Can you work these out from the model? Positions are in its coordinate system, mm. Round coordinates to 2 decimals unless told otherwise and drop trailing zeros. Order: outer loops, then holes, each group sorted by start corner. A loop starts at its lowest first (then second) coordinate and runs counter-clockwise, first axis right, second up. Notation, with made-up numbers: (64, 78) - (106, 78) arc R16 cw to (106, 99) - close; hole circle Ø10 at (34, 35.5). An arc over 180 degrees is marked (long way). Write item = value, one per line.
from build123d import *

# Parameters (mm, degrees)
ESBO_O1_W                = 250
ESBO_O1_H                = 130
RESSALTO_EXTRUS_O1_DEPTH = 6
FILETE1_R                = 50
ESBO_O2_R                = 2
CORTE_EXTRUS_O1_DEPTH    = 6
ESBO_O3_R                = 2.1
CORTE_EXTRUS_O2_DEPTH    = 6
ESBO_O4_R                = 2
CORTE_EXTRUS_O3_DEPTH    = 6
CHANFRO1_SIZE            = 2.3


with BuildPart() as part:
    # Esboço1 → Ressalto-extrusão1 (new body)
    with BuildSketch(Plane.XY):
        Rectangle(ESBO_O1_W, ESBO_O1_H)
    extrude(amount=RESSALTO_EXTRUS_O1_DEPTH)

    # Filete1
    filete1_edges = [part.edges().sort_by_distance(p)[0] for p in [
        (-125, 65, 3),
    ]]
    fillet(filete1_edges, radius=FILETE1_R)

    # Esboço2 → Corte-extrusão1 (cut)
    with BuildSketch(Plane(origin=(0, 0, 0), x_dir=(-1, 0, 0), z_dir=(0, 0, -1))):
        with Locations((0, -55)):
            Circle(ESBO_O2_R)
        with Locations((105, -55)):
            Circle(ESBO_O2_R)
        with Locations((-105, -55)):
            Circle(ESBO_O2_R)
    extrude(amount=-CORTE_EXTRUS_O1_DEPTH, mode=Mode.SUBTRACT)

    # Esboço3 → Corte-extrusão2 (cut)
    with BuildSketch(Plane(origin=(0, 0, 0), x_dir=(-1, 0, 0), z_dir=(0, 0, -1))):
        with Locations((-70, 55)):
            Circle(ESBO_O3_R)
        with Locations((-70, 35)):
            Circle(ESBO_O3_R)
    extrude(amount=-CORTE_EXTRUS_O2_DEPTH, mode=Mode.SUBTRACT)

    # Esboço4 → Corte-extrusão3 (cut)
    with BuildSketch(Plane(origin=(0, 0, 0), x_dir=(-1, 0, 0), z_dir=(0, 0, -1))):
        with Locations((-70, 15)):
            Circle(ESBO_O4_R)
        with Locations((-70, -35)):
            Circle(ESBO_O4_R)
    extrude(amount=-CORTE_EXTRUS_O3_DEPTH, mode=Mode.SUBTRACT)

    # Chanfro1
    chanfro1_edges = [part.edges().sort_by_distance(p)[0] for p in [
        (-103, -55, 0),
        (2, -55, 0),
        (107, -55, 0),
        (72.1, 55, 0),
        (72.1, 35, 0),
        (72, 15, 0),
        (72, -35, 0),
    ]]
    chamfer(chanfro1_edges, length=CHANFRO1_SIZE)


solid = part.part
(1) If we section it at A-A (z = 4.5): Write out the boundary of the cut face in (x, y), plus the area to 3 significant figures.
Computed:
outline = (-125, -65) - (125, -65) - (125, 65) - (-75, 65) arc R50 ccw to (-125, 15) - close; hole circle Ø4 at (-105, -55); hole circle Ø4 at (0, -55); hole circle Ø4.2 at (70, 35); hole circle Ø4.2 at (70, 55); hole circle Ø4 at (70, -35); hole circle Ø4 at (70, 15); hole circle Ø4 at (105, -55)
area = 31,900 mm^2
(2) Thinking about a two-plate mould opening in X: for faces 1 (the face through (69.026, -36.873, 2.188)), 2 (the face through (-110.742, 49.964, 3.042)), 3 (the face through (125, -1, 3)), which applies, +X half, -X half, draft (parallel to the pull), parting line (faces both ways), or undercut?
Computed:
face_1 = undercut
face_2 = -X half
face_3 = +X half
(3) Will these pins go through, and if not, where does the flat tip stop? P1, Ø4, axis at x = 70, y = 55, coming from the -Z side; P2, Ø6.5, axis at x = 70, y = 35, coming from the -Z side.
Computed:
P1 = through
P2 = 1.15
(4) If I drill on line 1 (Y direction, x = 70, z = 3.95); line 2 (X direction, y = 55, z = 1.5); line 3 (Y direction, x = -105, z = 3.7), over which ranges is the centre line in solid material (lowest first)? Write a range as from..to.
Computed:
line_1 = -65..-37, -33..13, 17..32.9, 37.1..52.9, 57.1..65
line_2 = -105..67.1, 72.9..125
line_3 = -65..-57, -53..55
